```python
from build123d import *

# Parameters (mm, degrees)
SKETCH1_W           = 29.2
SKETCH1_H           = 11
SKETCH1_R           = 1
BOSS_EXTRUDE1_DEPTH = 13.2
SKETCH6_R           = 1.85
CUT_EXTRUDE3_DEPTH  = 11.5
BOSS_EXTRUDE4_DEPTH = 2.5
SKETCH8_R           = 1.85
BOSS_EXTRUDE5_DEPTH = 3


with BuildPart() as part:
    # Sketch1 → Boss-Extrude1 (new body)
    with BuildSketch(Plane.XY):
        with Locations((14.6, 5.5)):
            Rectangle(SKETCH1_W, SKETCH1_H)
        with Locations((7.5, 8.2)):
            Circle(SKETCH1_R, mode=Mode.SUBTRACT)
    extrude(amount=BOSS_EXTRUDE1_DEPTH)

    # Sketch6 → Cut-Extrude3 (cut)
    with BuildSketch(Plane(origin=(0, 0, 0), x_dir=(-1, 0, 0), z_dir=(0, 0, -1))):
        with Locations((-7.5, 8.2)):
            Circle(SKETCH6_R)
    extrude(amount=-CUT_EXTRUDE3_DEPTH, mode=Mode.SUBTRACT)

    # Sketch7 → Boss-Extrude4 (add)
    with BuildSketch(Plane(origin=(0, 0, 0), x_dir=(-1, 0, 0), z_dir=(0, 0, -1))):
        Polygon((-20.1, 11), (-10.7, 11), (-9.2, 12.5), (-9.2, 17.25), (0, 17.25), (0, 22.25), (-29.2, 22.25), (-29.2, 17.25), (-21.6, 17.25), (-21.6, 12.5), align=None)
    extrude(amount=-BOSS_EXTRUDE4_DEPTH)

    # Sketch8 → Boss-Extrude5 (add)
    with BuildSketch(Plane(origin=(0, 0, 0), x_dir=(-1, 0, 0), z_dir=(0, 0, -1))):
        Polygon((-29.2, 22.25), (0, 22.25), (0, 16), (0, 10.75), (0, 0), (-29.2, 0), (-29.2, 10.75), (-29.2, 16), align=None)
        with Locations((-7.5, 8.2)):
            Circle(SKETCH8_R, mode=Mode.SUBTRACT)
        with Locations((-6.15, 14.5)):
            Circle(SKETCH8_R, mode=Mode.SUBTRACT)
    extrude(amount=BOSS_EXTRUDE5_DEPTH)


solid = part.part
```
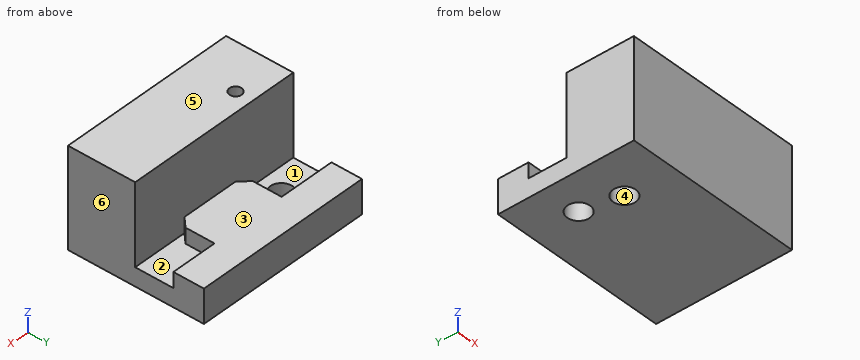
Input: part model. Units: mm. Frame: model coordinates. Face numbers are marked on the shaded views. A direction names the side the tool comes from. Round coordinates to 2 decimals unless told otherwise and drop trailing zeros. Loops run counter-clockwise (first coordinate to the right, second up) from the corner with the lowest first, then second, coordinate; pieces in that order, holes last. Notation, with made-up numbers: (2.25, 81) -> (45.25, 81) arc R24 cw to (45.25, 116) -> close; hole circle Ø11 at (83, 46). An arc over 180 degrees is marked (long way). One line per item, written item: value.
(1) Section A-A (y = 14.5). Return the cut outline in (x, z).
Geometry check:
outline: (0, -3) -> (4.3, -3) -> (4.3, 0) -> (0, 0) -> close; (8, -3) -> (29.2, -3) -> (29.2, 0) -> (21.6, 0) -> (21.6, 2.5) -> (9.2, 2.5) -> (9.2, 0) -> (8, 0) -> close
(2) Mould query, pull axis X, two halves, no side actions, for the marked faces 4, 5 and 6. Classes: pulls with the +X half, pulls with the -X half, needs draft (parallel to the pull), parting line crosses it, or undercut.
Geometry check:
face 4: undercut
face 5: needs draft
face 6: pulls with the +X half
(3) Section C-C (x = 21). Return the cut outline in (y, z), plus the area to 3 significant figures.
Geometry check:
outline: (0, -3) -> (22.25, -3) -> (22.25, 2.5) -> (11.9, 2.5) -> (11.9, 0) -> (11, 0) -> (11, 13.2) -> (0, 13.2) -> close
area: 238 mm2
(4) Pin query (flat end, axial travel): pin 1 (3.5 mm diameter, centred on x = 14.5, y = 14.5, fed in from +Z); pin 2 (1 mm diameter, centred on y = 6, z = 2, fed in from -X); pin 3 (1.2 mm diameter, centred on y = 14.5, z = 1.5, fed in from -X); pin 4 (6 mm diameter, centred on x = 8, z = 9, fed in from +Y). Return the tip coordinate at first contact, or that it passes through.
Geometry check:
pin 1: z = 2.5
pin 2: x = 0
pin 3: x = 9.2
pin 4: y = 11
(5) Set-up query: the marked faces 1, 2 and 3. Return all of +Z, -Z, +X, -X, +Y, -Y with unobstructed straight access to the full face (end or side cutting, diameter ignored); none if empty.
Geometry check:
face 1: +Z, -X
face 2: +Z, +X
face 3: +Z, +X, -X, +Y
(6) Section B-B (z = -1.5). Return the cut outline in (x, y), plus the area to 3 significant figures.
Geometry check:
outline: (0, 0) -> (29.2, 0) -> (29.2, 22.25) -> (0, 22.25) -> close; hole circle Ø3.7 at (6.15, 14.5); hole circle Ø3.7 at (7.5, 8.2)
area: 628 mm2
(7) Section D-D (x = 4.75). Return the cut outline in (y, z).
Geometry check:
outline: (0, -3) -> (13.29, -3) -> (13.29, 0) -> (11, 0) -> (11, 13.2) -> (0, 13.2) -> close; (15.71, -3) -> (22.25, -3) -> (22.25, 2.5) -> (17.25, 2.5) -> (17.25, 0) -> (15.71, 0) -> close
(8) Material intervals for line 1 (X direction, y = 8.2, z = 12.35); line 2 (Y direction, x = 6.15, z = -1.05); line 3 (Y direction, x = 7.5, z = 4), sorted ascending. Write a range as [from, to].
Geometry check:
line 1: [0, 6.5], [8.5, 29.2]
line 2: [0, 6.94], [9.46, 12.65], [16.35, 22.25]
line 3: [0, 6.35], [10.05, 11]
